Geometry: final body of the model. Coordinates: model frame, mm. A direction names the side the tool comes from. Give positions to 0.01 mm unless a question says otherwise; leave off trailing zeros. Loops run counter-clockwise (first coordinate to the right, second up) from the corner with the lowest first, then second, coordinate; pieces in that order, holes last. Notation, with made-up numbers: (-13, 19) -> (26, 19) arc R19 cw to (26, 41) -> close; hole circle Ø6 at (37, -3). An arc over 180 degrees is marked (long way). One line per question, with ' | ' between items. Start each with the question number.
Item 1: Pin query (flat end, axial travel): P1, Ø11.5, axis at x = 47.5, y = -22.5, coming from the +Z side; P2, Ø10, axis at x = 36, y = -30, coming from the -Z side; P3, Ø7.5, axis at x = 63, y = -29.5, coming from the +Z side. Return the tip coordinate at first contact, or that it passes through.
Item 2: Mould query, pull axis X, two halves, no side actions, for faces 4 (the flat face through (67, -35.299, 30)), 5 (the flat face through (58.481, -25, 21)), 6 (the flat face through (76.193, -25, 18)). Classes: released by +X, released by -X, zero draft, split by the parting line, or undercut.
Item 3: Section A-A on z = 18. Return loops of the section in (x, y), then the cut area to 3 significant figures.
Item 4: Section B-B on y = -3. Return loops of the section in (x, z), then the cut area to 3 significant figures.
Item 5: Set-up query: faces 1 (the flat face through (38, -25, 0)), 2 (the flat face through (39, -25, 15.116)), 3 (the flat face through (67, -19.853, 30)). Return all of +Z, -Z, +X, -X, +Y, -Y with unobstructed straight access to the full face (end or side cutting, diameter ignored); none if empty.
Item 6: Material intervals for line 1 along X through (y, z) = (-15, 19); line 2 along Z through (x, y) = (42, -15); line 3 along X through (y, z) = (-27.5, 28), sorted ascending. Write a range as [from, to].
Item 7: Section C-C on z = 30. Return loops of the section in (x, y).
Item 8: Section D-D on x = 42. Return loops of the section in (y, z).
from build123d import *

# Parameters (mm, degrees)
F1_DEPTH = 25.4
F2_DEPTH = 25.4
F3_W     = 17.7121385932
F3_H     = 15.4453162104
F4_DEPTH = 12.7


with BuildPart() as f1:
    # F0 (on Front) → F1 (new body)
    with BuildSketch(Plane.XZ):
        Polygon((0, 35.8823463321), (0, 0), (76.1927291751, 0), (76.1927291751, 35.8823463321), (58.4805905819, 35.8823463321), (58.4805905819, 15.1163935661), (19.6971185505, 15.1163935661), (19.6971185505, 35.8823463321), align=None)
    extrude(amount=F1_DEPTH)

    # F2 (add): a face of the model
    f2_faces = [f1.faces().sort_by_distance(p)[0] for p in [
        (37.6819042915, -25.4, 14.7848969887),
    ]]
    extrude(f2_faces, amount=F2_DEPTH)

    # F3 (on face) → F4 (cut, symmetric)
    with BuildSketch(Plane.XY.offset(35.8823463321)):
        with Locations((67.3366598785, -27.5759203359)):
            Rectangle(F3_W, F3_H)
    extrude(amount=F4_DEPTH, both=True, mode=Mode.SUBTRACT)


solid = f1.part
Result sheet:
1) P1: stops at z = 15.12 | P2: stops at z = 0 | P3: stops at z = 23.18
2) face 4: zero draft | face 5: undercut | face 6: released by +X
3) outline: (0, -50.8) -> (19.7, -50.8) -> (19.7, 0) -> (0, 0) -> close; (58.48, -50.8) -> (76.19, -50.8) -> (76.19, 0) -> (58.48, 0) -> close | area: 1,900 mm²
4) outline: (0, 0) -> (76.19, 0) -> (76.19, 35.88) -> (58.48, 35.88) -> (58.48, 15.12) -> (19.7, 15.12) -> (19.7, 35.88) -> (0, 35.88) -> close | area: 1,930 mm²
5) face 1: -Z, +X, -X, +Y, -Y | face 2: +Z, +Y, -Y | face 3: +Z, +X
6) line 1: x = [0, 19.7], [58.48, 76.19] | line 2: z = [0, 15.12] | line 3: x = [0, 19.7]
7) outline: (0, -50.8) -> (19.7, -50.8) -> (19.7, 0) -> (0, 0) -> close; (58.48, -50.8) -> (76.19, -50.8) -> (76.19, -35.3) -> (58.48, -35.3) -> close; (58.48, -19.85) -> (76.19, -19.85) -> (76.19, 0) -> (58.48, 0) -> close
8) outline: (-50.8, 0) -> (0, 0) -> (0, 15.12) -> (-50.8, 15.12) -> close
